Verification items for the finished model (mm, model axes). Coordinates: 2 decimals unless noted, no trailing zeros. Order: outer loops, then holes, each group sorted by start corner. A loop starts at its lowest first (then second) coordinate and runs counter-clockwise, first axis right, second up. Notation, with made-up numbers: M 26,-14 L 37,-14 A13 ccw 37,8 Z; hole C 39.5,-29.5 d9. An arc over 180 degrees is marked long. Return JSON: item names as keys, results as strings. Group by question number.
Q1. Section check A-A, the plane x = 0. Enter the section's corners in (y, z).
Q2. Go/stop test with flat-tipped pins: pin 1 Ø10 at (x, z) = (-27.5, -21.5) entering from -Y; pin 2 Ø18 at (x, z) = (0, 0) entering from +Y; pin 3 Ø1.9 at (y, z) = (3, -112.5) entering from +X. Record where each tip stops, or that it passes through.
Q3. Section check D-D, the plane x = 25. Enter the section's corners in (y, z), then the cut area to 3 significant figures.
Q4. Section check C-C, the plane y = 2.25. Count the separate pieces of the cut face and the enclosed holes in it, then the cut area to 3 significant figures.
Q5. Section check B-B, the plane z = 0. Enter the section's corners in (x, y), then the cut area to 3 significant figures.
Q6. Mould release check, pull along X, two halves, no side actions. Record for faces 1 (the face through (-26, 0, -2)), 2 (the face through (-43.548, 3.131, -97.586)), 3 (the face through (62, 3.1, 95.2)): pulls with the +X half, pulls with the -X half, needs draft (parallel to the pull), parting line crosses it, or undercut.
Q7. Thickness scan on probe 1 along X at (y, z) = (4, 33); probe 2 along X at (y, z) = (2.75, -4); probe 3 along Z at (x, y) = (-45, 4.5). Record the ranges inside material, lowest first.
from build123d import *

# Parameters (mm, degrees)
SKETCH1_R           = 125
SKETCH1_R_2         = 25.4
SKETCH1_R_3         = 10
SKETCH1_W           = 12.5
SKETCH1_H           = 12.5
BOSS_EXTRUDE1_DEPTH = 6.35


with BuildPart() as part:
    # Sketch1 → Boss-Extrude1 (new body)
    with BuildSketch(Plane(origin=(0, 0, 0), x_dir=(1, 0, 0), z_dir=(0, 1, 0))):
        with Locations(Location((0, 0, 0), (0, 0, 270))):
            Circle(SKETCH1_R)
        with Locations(Location((11.46043037, 53.917085788, 0), (0, 0, 270))):
            Circle(SKETCH1_R_2, mode=Mode.SUBTRACT)
        with Locations(Location((40.963350806, -36.883566733, 0), (0, 0, 270))):
            Circle(SKETCH1_R_2, mode=Mode.SUBTRACT)
        with Locations(Location((-52.423781176, -17.033519055, 0), (0, 0, 270))):
            Circle(SKETCH1_R_2, mode=Mode.SUBTRACT)
        with Locations(Location((0, 0, 0), (0, 0, 270))):
            Circle(SKETCH1_R_3, mode=Mode.SUBTRACT)
        Polygon((42.983091671, 111.786574462), (37.898883633, 100.367256242), (49.318201853, 95.283048203), (54.402409892, 106.702366424), align=None, mode=Mode.SUBTRACT)
        with Locations((0.048751666, 113.22779336)):
            Rectangle(SKETCH1_W, SKETCH1_H, mode=Mode.SUBTRACT)
        Polygon((84.786921515, 84.755223028), (75.497611197, 76.391090449), (83.861743776, 67.10178013), (93.151054095, 75.46591271), align=None, mode=Mode.SUBTRACT)
        Polygon((119.865992309, -6.096099115), (107.434468617, -4.789493325), (106.127862826, -17.221017017), (118.559386518, -18.527622808), align=None, mode=Mode.SUBTRACT)
        Polygon((107.075743235, -54.207050868), (96.250425688, -47.957050868), (90.000425688, -58.782368416), (100.825743235, -65.032368416), align=None, mode=Mode.SUBTRACT)
        Polygon((75.82278228, -92.956329333), (68.475466627, -82.843616903), (58.362754197, -90.190932557), (65.710069851, -100.303644987), align=None, mode=Mode.SUBTRACT)
        Polygon((31.511030318, -115.643832236), (28.912134183, -103.416987227), (16.685289174, -106.015883362), (19.284185309, -118.242728371), align=None, mode=Mode.SUBTRACT)
        Polygon((-64.708058023, -100.597537613), (-57.360742369, -90.484825183), (-67.473454799, -83.137509529), (-74.820770452, -93.250221959), align=None, mode=Mode.SUBTRACT)
        Polygon((-99.978239904, -65.465381118), (-89.152922357, -59.215381118), (-95.402922357, -48.39006357), (-106.228239904, -54.64006357), align=None, mode=Mode.SUBTRACT)
        Polygon((-117.909618955, -19.024883755), (-105.478095263, -17.718277964), (-106.784701054, -5.286754272), (-119.216224746, -6.593360063), align=None, mode=Mode.SUBTRACT)
        Polygon((-115.401696837, 30.693970582), (-103.513490383, 26.831258152), (-99.650777953, 38.719464606), (-111.538984407, 42.582177036), align=None, mode=Mode.SUBTRACT)
        Polygon((-54.26167929, 106.498998102), (-49.177471251, 95.079679882), (-37.758153031, 100.16388792), (-42.842361069, 111.583206141), align=None, mode=Mode.SUBTRACT)
    extrude(amount=BOSS_EXTRUDE1_DEPTH)


solid = part.part
Numbers:
{
 "1": {"outline": "M 0,-125 L 6.35,-125 L 6.35,-119.48 L 0,-119.48 Z; M 0,-106.98 L 6.35,-106.98 L 6.35,-76.58 L 0,-76.58 Z; M 0,-31.25 L 6.35,-31.25 L 6.35,-10 L 0,-10 Z; M 0,10 L 6.35,10 L 6.35,125 L 0,125 Z"},
 "2": {"pin 1": "stops at y = 0", "pin 2": "passes through", "pin 3": "stops at x = 56.41"},
 "3": {"outline": "M 0,-122.47 L 6.35,-122.47 L 6.35,-75.41 L 0,-75.41 Z; M 0,-32.43 L 6.35,-32.43 L 6.35,17.13 L 0,17.13 Z; M 0,56.64 L 6.35,56.64 L 6.35,104.25 L 0,104.25 Z; M 0,117.03 L 6.35,117.03 L 6.35,122.47 L 0,122.47 Z", "area": "950 mm2"},
 "4": {"separate pieces": "1", "enclosed holes": "16", "area": "40,800 mm2"},
 "5": {"outline": "M -125,0 L -71.27,0 L -71.27,6.35 L -125,6.35 Z; M -33.58,0 L -10,0 L -10,6.35 L -33.58,6.35 Z; M 10,0 L 125,0 L 125,6.35 L 10,6.35 Z", "area": "1,220 mm2"},
 "6": {"face 1": "needs draft", "face 2": "undercut", "face 3": "undercut"},
 "7": {"probe 1": "x = -120.57 to -72.18, -32.67 to 15.86, 66.06 to 120.57", "probe 2": "x = -124.94 to -66.66, -38.18 to -9.17, 9.17 to 124.94", "probe 3": "z = -116.62 to -110.62, -96.94 to -7.26, 41.32 to 116.62"}
}
